Here's how the part is built. I have some questions about the finished solid (model axes, mm). Face numbers are marked on the shaded views. Round coordinates to 2 decimals unless told otherwise and drop trailing zeros. Loops run counter-clockwise (first coordinate to the right, second up) from the corner with the lowest first, then second, coordinate; pieces in that order, holes last. Notation, with made-up numbers: M 11.25,-17.5 L 23.25,-17.5 A37 ccw 23.25,18.5 Z; hole C 20.5,1.5 d10. An arc over 180 degrees is marked long. Put each result on its own line as item: value. Start each with the question number.
```python
from build123d import *

# Parameters (mm, degrees)
SKETCH1_R           = 156
BOSS_EXTRUDE1_DEPTH = 400
SKETCH2_W           = 25
SKETCH2_H           = 100
BOSS_EXTRUDE2_DEPTH = 150
SKETCH3_R           = 13
CUT_EXTRUDE1_DEPTH  = 462.224728305
FILLET1_R           = 40
FILLET3_R           = 20
FILLET4_R           = 50
SHELL1_T            = -15


with BuildPart() as part:
    # Sketch1 → Boss-Extrude1 (new body)
    with BuildSketch(Plane.XY):
        Circle(SKETCH1_R)
    extrude(amount=BOSS_EXTRUDE1_DEPTH)

    # Sketch2 → Boss-Extrude2 (add)
    with BuildSketch(Plane(origin=(0, 0, 0), x_dir=(-1, 0, 0), z_dir=(0, 0, -1))):
        Rectangle(SKETCH2_W, SKETCH2_H)
    extrude(amount=BOSS_EXTRUDE2_DEPTH)

    # Sketch3 → Cut-Extrude1 (cut, through all)
    with BuildSketch(Plane(origin=(12.5, 0, 0), x_dir=(0, 0, -1), z_dir=(1, 0, 0))):
        with Locations((112, 0)):
            Circle(SKETCH3_R)
    extrude(amount=-CUT_EXTRUDE1_DEPTH, mode=Mode.SUBTRACT)

    # Fillet1
    fillet1_edges = [part.edges().sort_by_distance(p)[0] for p in [
        (0, 50, -150),
        (0, -50, -150),
    ]]
    fillet(fillet1_edges, radius=FILLET1_R)

    # Fillet3
    fillet3_edges = [part.edges().sort_by_distance(p)[0] for p in [
        (12.5, 0, 0),
        (0, -50, 0),
        (-12.5, 0, 0),
        (0, 50, 0),
    ]]
    fillet(fillet3_edges, radius=FILLET3_R)

    # Fillet4
    fillet4_edges = [part.edges().sort_by_distance(p)[0] for p in [
        (-156, 0, 0),
    ]]
    fillet(fillet4_edges, radius=FILLET4_R)

    # Shell1
    shell1_openings = [part.faces().sort_by_distance(p)[0] for p in [
        (0, 0, 400),
    ]]
    offset(amount=SHELL1_T, openings=shell1_openings)


solid = part.part
```
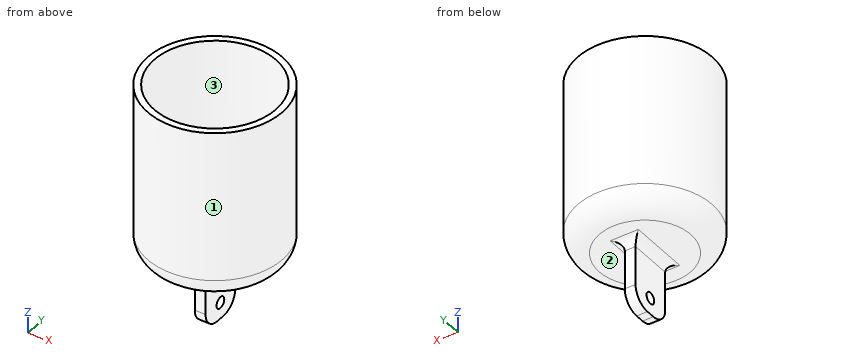
1) If I drill on probe 1 along Y at (x, z) = (0, 197); probe 2 along Y at (x, z) = (-2.75, -112); probe 3 along Z at (x, y) = (-78, 31), over which ranges is the centre line in solid material (lowest first)? Write a range as from..to.
2) I'm going to push flat-ended pins straight in: P1, Ø1, axis at x = 90, y = 10, coming from the -Z side; P2, Ø8, axis at x = 94, z = 317, coming from the -Y side; P3, Ø2, axis at y = 77, z = 98, coming from the -X side. Where does each tip first touch, or does it pass through?
3) If we mould it in two halves opening along Y, with no side actions, what happens to the marked faces 1, 2 and 3? For each: pulls with the +Y half, pulls with the -Y half, needs draft (parallel to the pull), parting line crosses it, or undercut.
4) Suppose I cut it at A-A (y = 0). Write out the boundary of the cut face in (x, z).
5) Suppose I cut it at B-B (z = 255.5). Write out the boundary of the cut face in (x, y), plus the area to 3 significant figures.
Results are:
1. probe 1: -156..-141, 141..156
1. probe 2: -49.95..-13, 13..49.95
1. probe 3: 0..15
2. P1: z = 0
2. P2: y = -127.42
2. P3: x = -136.24
3. face 1: parting line crosses it
3. face 2: needs draft
3. face 3: undercut
4. outline: M -156,50 A50 ccw -106,0 L -32.5,0 A20 cw -12.5,-20 L -12.5,-99 L 12.5,-99 L 12.5,-20 A20 cw 32.5,0 L 106,0 A50 ccw 156,50 L 156,400 L 141,400 L 141,50 A35 cw 106,15 L 32.5,15 A35 ccw 0,-7.01 A35 ccw -32.5,15 L -106,15 A35 cw -141,50 L -141,400 L -156,400 Z; M -12.5,-150 L 12.5,-150 L 12.5,-125 L -12.5,-125 Z
5. outline: C 0,0 d312; hole C 0,0 d282
5. area: 14,000 mm²
